Autodesk Inventor part; units mm, degrees
ref_plane "YZ Plane" through (0, 0, 0) normal (1, 0, 0) x (0, 1, 0)
ref_plane "XZ Plane" through (0, 0, 0) normal (0, 1, 0) x (-1, 0, 0)
ref_plane "XY Plane" through (0, 0, 0) normal (0, 0, 1) x (1, 0, 0)
sketch "Sketch1" plane through (0, 0, 0) normal (0, 0, 1) x (1, 0, 0)
  line L0 (-30, -6) -> (30, -6)
  line L1 (30, -6) -> (30, 6)
  line L2 (30, 6) -> (-30, 6)
  line L3 (-30, 6) -> (-30, -6)
  line L4 (-30, -6) -> (30, 6) construction
  line L5 (30, -6) -> (-30, 6) construction
  line L6 (30, 6) -> (25, 6) construction
  line L7 (-30, 6) -> (-25, 6) construction
  point P0 (0, 0)
  dimension "d0" = 60
  dimension "d1" = 12
extrude "Block" add sketch "Sketch1" along normal blind 60
sketch "Sketch2" plane through (30, -6, 0) normal (1, 0, 0) x (0, 0, -1)
  line L0 (0, 12) -> (-60, 12)
  line L1 (-30, 12) -> (-15.25, 12)
  line L2 (-30, 12) -> (-44.75, 12)
  line L3 (-30, 12) -> (-30, 3.1) construction
  line L4 (-30, 3.1) -> (-8.25, 3.1)
  line L5 (-30, 3.1) -> (-51.75, 3.1)
  line L6 (-51.75, 3.1) -> (-51.75, 5.1)
  line L7 (-8.25, 3.1) -> (-8.25, 5.1)
  line L8 (-8.25, 5.1) -> (-15.25, 12)
  line L9 (-51.75, 5.1) -> (-44.75, 12)
  point P0 (0, 6)
  dimension "d17" = 14.75
  dimension "d18" = 14.75
  dimension "d19" = 8.9
  dimension "d20" = 21.75
  dimension "d21" = 21.75
  dimension "d22" = 2
  dimension "d23" = 2
extrude "Tripod Slot" cut sketch "Sketch2" against normal blind 60
hole "Hole1" at (0, -2.9, 30) direction (0, -1, 0) diameter 22.5 end through all
sketch "Sketch4" plane through (0, 0, 0) normal (0, 0, -1) x (-1, 0, 0)
  line L0 (-30, 6) -> (30, 6)
  line L1 (-12.7, -6) -> (12.7, -6)
  line L2 (12.7, -6) -> (12.7, 6)
  line L3 (12.7, 6) -> (-12.7, 6)
  line L4 (-12.7, 6) -> (-12.7, -6)
  line L5 (-12.7, -6) -> (12.7, 6) construction
  line L6 (12.7, -6) -> (-12.7, 6) construction
  point P0 (0, 0)
  dimension "d64" = 25.4
  dimension "d65" = 25.288
  dimension "d66" = 17.3
extrude "Extrusion4" add sketch "Sketch4" along normal blind 52.5
sketch "Sketch5" plane through (-30, 6, 15.25) normal (0, 1, 0) x (1, 0, 0)
  line L0 (60, -29.5) -> (60, 0)
  line L1 (17.3, 67.75) -> (42.7, 67.75)
  line L2 (42.7, 15.25) -> (42.7, 67.75)
  line L3 (17.3, 67.75) -> (42.7, 67.75)
  line L4 (42.7, 67.75) -> (42.7, 45.25)
  line L5 (42.7, 45.25) -> (17.3, 45.25)
  line L6 (17.3, 45.25) -> (17.3, 67.75)
  line L7 (17.3, 15.25) -> (17.3, 67.75) construction
  line L8 (42.7, 45.25) -> (17.3, 67.75) construction
  circle A0 centre (30, 56.5) radius 1.5
  point P0 (30, 15.25)
  dimension "d67" = 22.5
  dimension "d68" = 3
extrude "Extrusion5" add sketch "Sketch5" along normal blind 40
sketch "Sketch6" plane through (0, 0, -52.5) normal (0, 0, -1) x (-1, 0, 0)
  line L0 (0, 0) -> (0, 46) construction
  circle A0 centre (0, 36) radius 2.5
  line L1 (-12.7, 46) -> (12.7, 46) construction
  line L2 (-12.7, 46) -> (12.7, 46) construction
  line L3 (12.7, 46) -> (0, 46) construction
  line L4 (0, 36) -> (0, 46) construction
  dimension "d60" = 5
  dimension "d61" = 10
extrude "Extrusion6" cut sketch "Sketch6" against normal blind 31.75
fillet "Fillet4" radius 11 2 edges at (12.7, 46, -41.25) (-12.7, 46, -41.25)
fillet "Fillet5" radius 20 1 edges at (0, -6, -52.5)
fillet "Fillet6" radius 5 1 edges at (0, 6, -30)
sketch "Sketch7" plane through (0, 0, 60) normal (0, 0, 1) x (1, 0, 0)
  line L0 (-30, 6) -> (30, 6)
  line L1 (-12.7, -6) -> (12.7, -6)
  line L2 (12.7, -6) -> (12.7, 6)
  line L3 (12.7, 6) -> (-12.7, 6)
  line L4 (-12.7, 6) -> (-12.7, -6)
  line L5 (-12.7, -6) -> (12.7, 6) construction
  line L6 (12.7, -6) -> (-12.7, 6) construction
  point P0 (0, 0)
  dimension "d73" = 25.4
extrude "Extrusion7" add sketch "Sketch7" along normal blind 35
sketch "Sketch8" plane through (-30, 6, 44.75) normal (0, 1, 0) x (1, 0, 0)
  line L0 (30, -50.25) -> (30, 0) construction
  line L1 (60, 0) -> (0, 0) construction
  line L2 (30, -50.25) -> (30, -47.75) construction
  line L3 (17.3, -15.25) -> (17.3, -50.25)
  line L4 (42.7, -50.25) -> (17.3, -50.25)
  line L5 (17.3, -50.25) -> (17.3, -45.25)
  line L6 (17.3, -45.25) -> (42.7, -45.25)
  line L7 (42.7, -45.25) -> (42.7, -50.25)
  line L8 (42.7, -50.25) -> (17.3, -45.25) construction
  line L9 (17.3, -50.25) -> (42.7, -45.25) construction
  point P0 (30, 44.75)
  dimension "d76" = 2.5
  dimension "d81" = 5
extrude "Extrusion8" add sketch "Sketch8" along normal blind 40
hole "Hole2" at (0, 36, 95) direction (0, 0, -1) diameter 3 end through all
fillet "Fillet7" radius 12.7 2 edges at (12.7, 46, 92.5) (-12.7, 46, 92.5)
fillet "Fillet8" radius 5 1 edges at (0, 6, 90)
fillet "Fillet9" radius 5 1 edges at (0, -6, 95)
fillet "Fillet10" radius 7.5 4 edges at (12.7, 0, 0) (-12.7, 0, 0) (-12.7, 0, 60) (12.7, 0, 60)
fillet "Fillet11" radius 1.5 2 edges at (0, -6, 18.75) (0, -2.9, 18.75)
properties part number "InnerFrame"
Model file for the job. Use its own axes, mm. A direction names the side the tool comes from. Coordinates: 2 decimals unless noted, no trailing zeros. Write each loop counter-clockwise with the first axis right and the second up, starting at its lowest first coordinate (ties: lowest second). Pieces come first, ordered by that corner, then holes. Notation, with made-up numbers: (45, -2) - (71, -2) arc R20 cw to (71, 27) - close; hole circle Ø4 at (29.25, -38.75). An arc over 180 degrees is marked (long way). Write each question's results on one line, items separated by ' | '. Start each with the question number.
1) Cut at D-D (z = 12). Write the cut outline in (x, y).
2) Cut at A-A (z = 30). Write the cut outline in (x, y).
3) Probe line 1 along Z through (x, y) = (0, 14.75); line 2 along Z through (x, y) = (7.5, 23.5); line 3 along Y through (x, z) = (-2, -18). List the from-to ranges inside material, lowest first. Write a range as from..to.
4) Cut at B-B (y = 42.5). Write the cut outline in (x, z).
5) Cut at C-C (x = 25.5). Write the cut outline in (y, z), then the cut area to 3 significant figures.
6) Mould opens along Y. For faces 6 (the face through (14.955, 0.084, 62.139)), 7 (the face through (0.9, 37.2, 92.5)), 8 (the face through (13, -6, 28)) say: pulls with the +Y half, pulls with the -Y half, needs draft (parallel to the pull), parting line crosses it, or undercut.
7) Flat gauge pins, fed straight in: P1, Ø2.5, axis at x = 0, z = -41.25, coming from the +Y side; P2, Ø2, axis at x = -8.5, y = -2, coming from the -Z side; P3, Ø5, axis at x = 0, z = -41.25, coming from the -Y side. Where does each tip first touch, or does it go through?
8) 3-axis set-ups, long thin cutter, end or side, ignore diameter. For faces 1 (the face through (-12.7, 5, 84)), 2 (the face through (2.5, 36.1, -41.4)), 3 (the face through (0, 8, 89)), 4 (the face through (-8.88, 42.38, 92.54)), 5 (the face through (12.7, 5, 84)): which of +Z, -Z, +X, -X, +Y, -Y reach the whole face in a straight line?
Returned:
1) outline: (-30, -6) - (30, -6) - (30, -2.9) - (-30, -2.9) - close; (-30, 2.8) - (30, 2.8) - (30, 6) - (-30, 6) - close
2) outline: (-30, -6) - (-12.75, -6) arc R1.5 ccw to (-11.25, -4.5) - (-11.25, -4.4) arc R1.5 ccw to (-12.75, -2.9) - (-30, -2.9) - close; (11.25, -4.5) arc R1.5 ccw to (12.75, -6) - (30, -6) - (30, -2.9) - (12.75, -2.9) arc R1.5 ccw to (11.25, -4.4) - close
3) line 1: -52.5..-42.75, -39.75..-30, 90..95 | line 2: -52.5..-30, 90..95 | line 3: -6..6
4) outline: (-9.75, -52.5) - (9.75, -52.5) - (9.75, -30) - (-9.75, -30) - close; (-8.76, 90) - (8.76, 90) - (8.76, 95) - (-8.76, 95) - close; hole circle Ø3 at (0, -41.25)
5) outline: (-6, 0) - (6, 0) - (6, 15.25) - (-0.9, 8.25) - (-2.9, 8.25) - (-2.9, 51.75) - (-0.9, 51.75) - (6, 44.75) - (6, 60) - (-6, 60) - close | area: 381 mm^2
6) face 6: needs draft | face 7: undercut | face 8: pulls with the -Y half
7) P1: y = 6 | P2: z = -45.73 | P3: y = -5
8) face 1: +Z, -X, +Y, -Y | face 2: -Z | face 3: +X, -X, +Y | face 4: +Z, -X, +Y | face 5: +Z, +X, +Y, -Y
